Part model, mm, in its own coordinate system. A direction names the side the tool comes from. Give positions to 0.01 mm unless a question says otherwise; leave off trailing zeros. Order: outer loops, then holes, each group sorted by start corner. A loop starts at its lowest first (then second) coordinate and runs counter-clockwise, first axis right, second up.
1. Slice it at B-B on x = 0. Give the number of separate pieces and of enclosed holes in the cut face, and give its area (3 significant figures).
2. Which spindle directions (+Z, -Z, +X, -X, +Y, -Y) get a long thin tool onto all of the face, cutting with end or side? Do faces 4 (the flat face through (-6.65, 0, 39)), 5 (the flat face through (-9.65, 0, 39)). Say none if no direction does.
3. Mould opens along Z. For faces 1 (the flat face through (10, 0, 0)), 2 (the flat face through (10, -7.65, 39)), 3 (the cylindrical face through (17.94, 0.11, 34.62)) say: +Z half, -Z half, draft (parallel to the pull), parting line (faces both ways), or undercut.
4. Slice it at A-A on y = 2. List the corners of the cut face in (x, z).
5. Drop a flat-ended pin along its axis: pin 1 Ø3 at (x, z) = (0, 60) entering from +Y. Give the stop position or say it passes through.
6. Slice it at C-C on z = 10. List the corners of the cut face in (x, y).
7. Probe line 1 (Y direction, x = 1, z = 7.5); line 2 (X direction, y = 1.75, z = 10); line 3 (X direction, y = 5.4, z = 10). List the from-to ranges inside material, lowest first.
8. Slice it at D-D on x = 5.5. List the corners of the cut face in (y, z), and give its area (3 significant figures).
from build123d import *

# Parameters (mm, degrees)
SKETCH_2_W          = 19.3
SKETCH_2_H          = 15.3
SKETCH_2_W_2        = 13.3
SKETCH_2_H_2        = 9.3
EXTRUDE_1_DEPTH     = 80
SKETCH_3_R          = 1.75
CUT_EXTRUDE_1_DEPTH = 100
SKETCH_5_W          = 20
SKETCH_5_H          = 15.3
EXTRUDE_2_DEPTH     = 80
SKETCH_6_R          = 1.75
CUT_EXTRUDE_2_DEPTH = 100


with BuildPart() as part:
    # 草图2 → 凸台-拉伸1 (new body)
    with BuildSketch(Plane.XY):
        Rectangle(SKETCH_2_W, SKETCH_2_H)
        Rectangle(SKETCH_2_W_2, SKETCH_2_H_2, mode=Mode.SUBTRACT)
    extrude(amount=EXTRUDE_1_DEPTH)

    # 草图3 → 切除-拉伸1 (cut)
    with BuildSketch(Plane(origin=(0, 7.65, 0), x_dir=(1, 0, 0), z_dir=(0, 1, 0))):
        with Locations(Location((0, -10, 0), (0, 0, 270))):
            Circle(SKETCH_3_R)
        with Locations(Location((0, -35, 0), (0, 0, 270))):
            Circle(SKETCH_3_R)
        with Locations(Location((0, -60, 0), (0, 0, 270))):
            Circle(SKETCH_3_R)
    extrude(amount=-CUT_EXTRUDE_1_DEPTH, mode=Mode.SUBTRACT)

    # 草图5 → 凸台-拉伸2 (add)
    with BuildSketch(Plane(origin=(0, 0, 0), x_dir=(-1, 0, 0), z_dir=(0, 0, -1))):
        with Locations((-19.65, 0)):
            Rectangle(SKETCH_5_W, SKETCH_5_H)
    extrude(amount=-EXTRUDE_2_DEPTH)

    # 草图6 → 切除-拉伸2 (cut)
    with BuildSketch(Plane(origin=(0, 7.65, 0), x_dir=(1, 0, 0), z_dir=(0, 1, 0))):
        with Locations(Location((19.65, -10, 0), (0, 0, 270))):
            Circle(SKETCH_6_R)
        with Locations(Location((19.65, -35, 0), (0, 0, 270))):
            Circle(SKETCH_6_R)
        with Locations(Location((19.65, -60, 0), (0, 0, 270))):
            Circle(SKETCH_6_R)
    extrude(amount=-CUT_EXTRUDE_2_DEPTH, mode=Mode.SUBTRACT)


solid = part.part
Data:
1. separate pieces: 8
1. enclosed holes: 0
1. area: 417 mm2
2. face 4: +Z, -Z
2. face 5: +Z, -Z, -X, +Y, -Y
3. face 1: -Z half
3. face 2: draft
3. face 3: undercut
4. outline: (-9.65, 0) - (-6.65, 0) - (-6.65, 80) - (-9.65, 80) - close; (6.65, 0) - (29.65, 0) - (29.65, 80) - (6.65, 80) - close; hole circle Ø3.5 at (19.65, 10); hole circle Ø3.5 at (19.65, 35); hole circle Ø3.5 at (19.65, 60)
5. pin 1: passes through
6. outline: (-9.65, -7.65) - (-1.75, -7.65) - (-1.75, -4.65) - (-6.65, -4.65) - (-6.65, 4.65) - (-1.75, 4.65) - (-1.75, 7.65) - (-9.65, 7.65) - close; (1.75, -7.65) - (17.9, -7.65) - (17.9, 7.65) - (1.75, 7.65) - (1.75, 4.65) - (6.65, 4.65) - (6.65, -4.65) - (1.75, -4.65) - close; (21.4, -7.65) - (29.65, -7.65) - (29.65, 7.65) - (21.4, 7.65) - close
7. line 1: y = -7.65 to -4.65, 4.65 to 7.65
7. line 2: x = -9.65 to -6.65, 6.65 to 17.9, 21.4 to 29.65
7. line 3: x = -9.65 to -1.75, 1.75 to 17.9, 21.4 to 29.65
8. outline: (-7.65, 0) - (-4.65, 0) - (-4.65, 80) - (-7.65, 80) - close; (4.65, 0) - (7.65, 0) - (7.65, 80) - (4.65, 80) - close
8. area: 480 mm2
